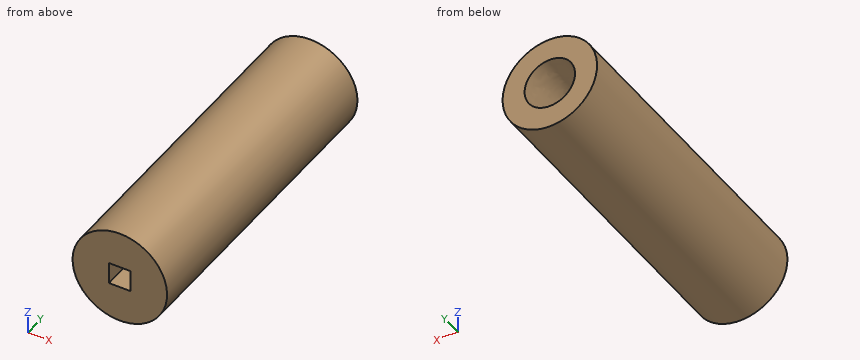
```python
from build123d import *

# Parameters (mm, degrees)
SKETCH1_R           = 7.5
BOSS_EXTRUDE1_DEPTH = 50
SKETCH3_W           = 3.45
SKETCH3_H           = 3.45
CUT_EXTRUDE2_DEPTH  = 25


with BuildPart() as part:
    # Sketch1 → Boss-Extrude1 (new body)
    with BuildSketch(Plane(origin=(0, 0, 0), x_dir=(1, 0, 0), z_dir=(0, 1, 0))):
        with Locations(Location((0, 0, 0), (0, 0, 270))):
            Circle(SKETCH1_R)
    extrude(amount=BOSS_EXTRUDE1_DEPTH)

    # Sketch3 → Cut-Extrude2 (cut)
    with BuildSketch(Plane.XZ):
        Rectangle(SKETCH3_W, SKETCH3_H)
    extrude(amount=-CUT_EXTRUDE2_DEPTH, mode=Mode.SUBTRACT)

    # Cut-Loft2: read off the stored shape, not the designer's step
    # Cut-Loft2: loft between two sections, ruled curve by curve
    cut_loft2_from = [
        Edge.make_bspline([(-1.423347069, 25, -0.473374188), (-2.370095445, 25, 2.373319949), (0.476598692, 25, 3.320068326), (1.423347069, 25, 0.473374188), (2.370095445, 25, -2.373319949), (-0.476598692, 25, -3.320068326), (-1.423347069, 25, -0.473374188)], [0, 0, 0, 0, 0.5, 0.5, 0.5, 1, 1, 1, 1], 3, [1, 0.333333333, 0.333333333, 1, 0.333333333, 0.333333333, 1]),
    ]
    cut_loft2_to = [
        Edge.make_bspline([(-3.971230311, 50, -0.478883932), (-4.928998175, 50, 7.463576689), (3.013462446, 50, 8.421344553), (3.971230311, 50, 0.478883932), (4.928998175, 50, -7.463576689), (-3.013462446, 50, -8.421344553), (-3.971230311, 50, -0.478883932)], [0, 0, 0, 0, 0.5, 0.5, 0.5, 1, 1, 1, 1], 3, [1, 0.333333333, 0.333333333, 1, 0.333333333, 0.333333333, 1]),
    ]
    cut_loft2 = Solid(Shell([*[Face.make_surface_from_curves(cut_loft2_from[k], cut_loft2_to[k]) for k in range(1)], Face(Wire(cut_loft2_from)), Face(Wire(cut_loft2_to))]))
    add(cut_loft2, mode=Mode.SUBTRACT)


solid = part.part
```
Check sheet for the modelled part. Datum: model origin and axes. Units: mm. Coordinates: 2 decimals unless noted, no trailing zeros. Loops run counter-clockwise (first coordinate to the right, second up) from the corner with the lowest first, then second, coordinate; pieces in that order, holes last.
1) Gauge pin test, flat ends, axial feed: pin 1 (4 mm diameter, centred on x = -2.5, y = 26, fed in from -Z); pin 2 (1 mm diameter, centred on y = 13.5, z = 4.5, fed in from +X); pin 3 (3 mm diameter, centred on x = 2.5, y = 26, fed in from -Z). Record the tip position at first contact, or that the pin passes through.
2) Sectioned sample at B-B (x = -4.5). Record the boundary of the cut face in (y, z), and give its area (3 significant figures).
3) Material ranges on probe 1 along X at (y, z) = (39, -0.75); probe 2 along X at (y, z) = (45.5, 2.5); probe 3 along Z at (x, y) = (0.75, 18.5) (3 decimals), recorded low to high.
4) Sectioned sample at C-C (z = 5.5). Record the boundary of the cut face in (x, y), and give its area (3 significant figures).
5) Sectioned sample at A-A (y = 3). Record the boundary of the cut face in (x, z) (3 decimals), and give its area (3 significant figures).
Check sheet entries:
1. pin 1: stops at z = -7.48
1. pin 2: stops at x = 6.34
1. pin 3: stops at z = -7.43
2. outline: (0, -6) - (50, -6) - (50, 6) - (0, 6) - close
2. area: 600 mm2
3. probe 1: x = -7.46 to -2.79, 2.79 to 7.46
3. probe 2: x = -7.07 to -2.51, 2.51 to 7.07
3. probe 3: z = -7.462 to -1.725, 1.725 to 7.462
4. outline: (-5.1, 0) - (5.1, 0) - (5.1, 50) - (-5.1, 50) - close
4. area: 510 mm2
5. outline: circle Ø15 at (0, 0); hole (-1.725, -1.725) - (1.725, -1.725) - (1.725, 1.725) - (-1.725, 1.725) - close
5. area: 165 mm2
